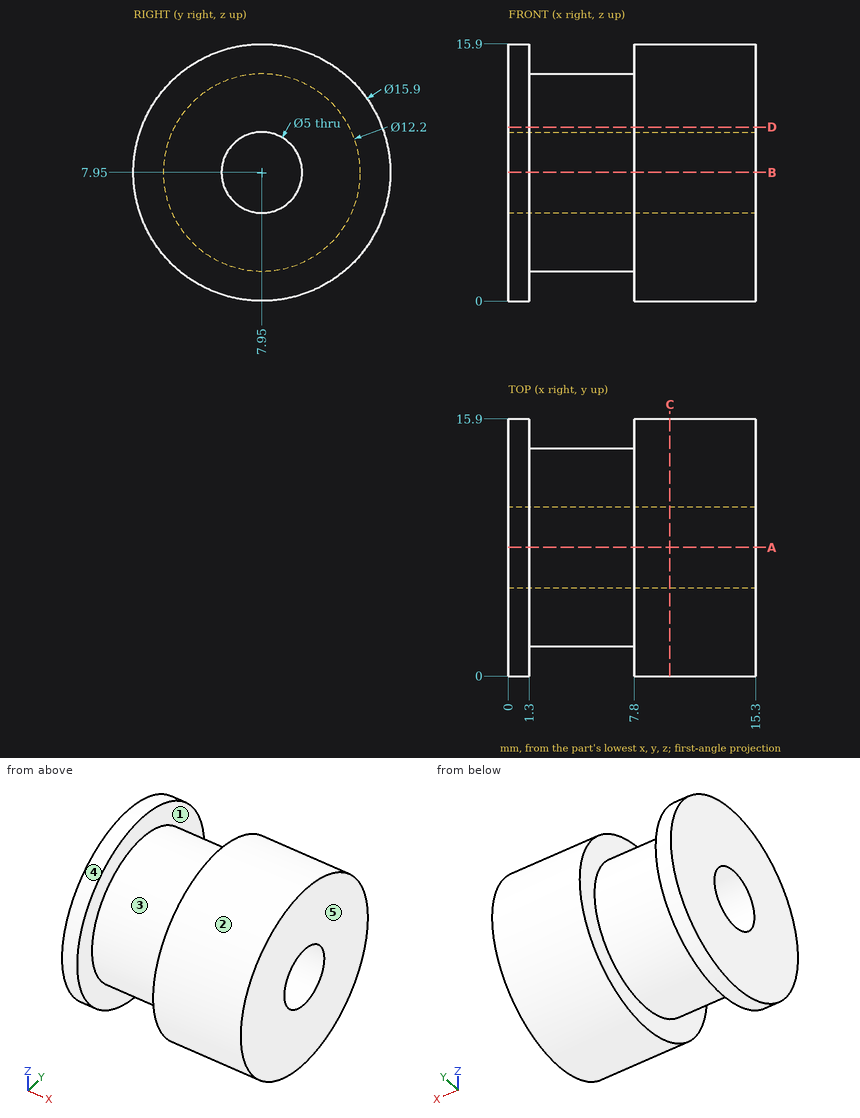
Geometry: see drawing. Coordinates: mm, zero at the bounding-box minimum. A direction names the side the tool comes from. Give positions to 0.01 mm unless a question says otherwise; leave off trailing zeros. Loops run counter-clockwise (first coordinate to the right, second up) from the corner with the lowest first, then second, coordinate; pieces in that order, holes last. Notation, with made-up numbers: (89, 16.5) - (137, 16.5) arc R24 ccw to (137, 50.5) - close; hole circle Ø4 at (-39.75, -31). An arc over 180 degrees is marked (long way). Answer as CSV lines item,"result". Start each with the question number.
1. Section D-D, the plane z = 10.75. Return loops of the section in (x, y).
2. Ray query, L1, parallel to Z at x = 10, y = 7.95; L2, parallel to X at y = 4.75, z = 13.25. Return the intervals inside material, ascending.
3. Pin query (flat end, axial travel): P1, Ø1, axis at x = 5.5, z = 8, coming from the +Y side; P2, Ø6, axis at x = 13.5, y = 14, coming from the +Z side; P3, Ø6, axis at x = 7.5, y = 2.5, coming from the -Z side. Return the tip coordinate at first contact, or that it passes through.
4. Section A-A, the plane y = 7.95. Return loops of the section in (x, z).
5. Reachability of the marked faces 1 and 2 from +Z, -Z, +X, -X, +Y, -Y: full face, straight path, thin tool, end or side. Return the list, or none.
6. Draft query along X for the marked faces 3, 4 and 5. Return one class per face: released by +X, released by -X, zero draft, split by the parting line, or undercut.
7. Section C-C, the plane x = 10. Return loops of the section in (y, z).
Answers:
1,outline,"(0, 0.51) - (1.3, 0.51) - (1.3, 2.53) - (7.8, 2.53) - (7.8, 0.51) - (15.3, 0.51) - (15.3, 15.39) - (7.8, 15.39) - (7.8, 13.37) - (1.3, 13.37) - (1.3, 15.39) - (0, 15.39) - close"
2,L1,"z = 0 to 5.45, 10.45 to 15.9"
2,L2,"x = 0 to 1.3, 7.8 to 15.3"
3,P1,"stops at y = 14.05"
3,P2,"stops at z = 15.29"
3,P3,"stops at z = 0.39"
4,outline,"(0, 0) - (1.3, 0) - (1.3, 1.85) - (7.8, 1.85) - (7.8, 0) - (15.3, 0) - (15.3, 5.45) - (0, 5.45) - close; (0, 10.45) - (15.3, 10.45) - (15.3, 15.9) - (7.8, 15.9) - (7.8, 14.05) - (1.3, 14.05) - (1.3, 15.9) - (0, 15.9) - close"
5,face 1,"none"
5,face 2,"+X, -X"
6,face 3,"undercut"
6,face 4,"zero draft"
6,face 5,"released by +X"
7,outline,"circle Ø15.9 at (7.95, 7.95); hole circle Ø5 at (7.95, 7.95)"
